The listing builds one solid part. Answer for the finished solid, in the listing's coordinates (mm). A direction names the side the tool comes from. Round coordinates to 2 decimals unless told otherwise and drop trailing zeros. Write each loop counter-clockwise with the first axis right and the second up, starting at its lowest first coordinate (ties: lowest second). Pieces come first, ordered by that corner, then holes. Notation, with made-up numbers: (-36, 32) - (-21, 32) arc R21 ccw to (-21, 46) - close; hole circle Ø1 at (70, 23). An arc over 180 degrees is marked (long way). Answer as CSV lines item,"result". Start each with the question number.
Item 1: Which of the six approach directions +Z, -Z, +X, -X, +Y, -Y give full straight-line access (tool end or side, diameter ignored) to faces 4 (the cylindrical face through (-0.54, 3.37, 2.44)), 5 (the flat face through (-1.293, -1.958, 0.76)), 6 (the flat face through (2, -3.1, 0))?
Item 2: Flat-ended cylindrical pins translate along their axes: pin 1 (5 mm diameter, centred on y = 2, z = 0, fed in from -X); pin 2 (1.5 mm diameter, centred on y = 2.5, z = 1, fed in from +X); pin 3 (4 mm diameter, centred on x = -3, y = 0, fed in from -Z). Find the tip coordinate at first contact, or state that the pin passes through.
Item 3: A cutting plane is placed at B-B on y = -0.5. Determine the outline of the cut face in (x, z).
Item 4: Straight lines are drawn through the part: line 1 along Z through (x, y) = (0, -1.5); line 2 along Y through (x, z) = (0.25, 2.25); line 3 along Z through (x, y) = (1.25, -1). For each, find the intervals that lie inside material, in ascending order. Write a range as [from, to].
Item 5: For a pull along Z with two mould halves and no side action, classify faces 1 (the flat face through (0, -2, -1.5)), 2 (the flat face through (0, 6.9, 0)), 3 (the conical face through (-0.351, -0.193, 2.671)) as pulls with the +Z half, pulls with the -Z half, needs draft (parallel to the pull), parting line crosses it, or undercut.
Item 6: A cutting plane is placed at A-A on y = 3.75. Determine the outline of the cut face in (x, z).
Solid Edge part; units mm, degrees
sketch "Sketch1" plane through (0, 0, 0) normal (0, 0, 1) x (1, 0, 0)
  line L0 (2.5, 0) -> (2.5, 6.9)
  line L1 (0, 6.9) -> (2.5, 6.9)
  line L2 (0, 0) -> (0, 6.9)
  line L3 (0, 0) -> (0, -3.1)
  line L4 (0, -3.1) -> (4.715, -3.1)
  line L5 (4.715, -3.1) -> (4.715, -2.215)
  line L6 (4.715, -2.215) -> (2.5, 0)
revolve "RevolvedProtrusion1" add sketch "Sketch1" angle 360 about axis through (0, 0, 0) along (0, 1, 0)
sketch "Sketch2" plane through (0, 0, 0) normal (1, 0, 0) x (0, 1, 0)
  line L0 (-3.1, 2.2215) -> (-1.2, 2.2215)
  line L1 (0.0826, 0) -> (-1.2, 2.2215)
  line L2 (-3.1, 0) -> (0.0826, 0)
  line L3 (-3.1, 0) -> (-3.1, 2.2215)
revolve "RevolvedCutout1" cut sketch "Sketch2" angle 360 about axis through (0, -4.5, 0) along (0, 1, 0)
sketch "Sketch3" plane through (0, -3.1, 0) normal (0, -1, 0) x (0, 0, 1)
  circle A0 centre (0, 0) radius 2.2215
  line L0 (-1.5, -0.866) -> (0, -1.7321)
  line L1 (0, -1.7321) -> (1.5, -0.866)
  line L2 (1.5, -0.866) -> (1.5, 0.866)
  line L3 (1.5, 0.866) -> (0, 1.7321)
  line L4 (0, 1.7321) -> (-1.5, 0.866)
  line L5 (-1.5, 0.866) -> (-1.5, -0.866)
extrude "Protrusion1" add sketch "Sketch3" against normal up to next
sketch "Sketch4" plane through (0, 0, 0) normal (0, 0, 1) x (1, 0, 0)
  line L0 (-1.7321, -3.1) -> (0, -3.1)
  line L1 (0, -3.1) -> (0, -2.6359)
  line L2 (0, -2.6359) -> (-1.7321, -3.1)
revolve "RevolvedCutout2" cut sketch "Sketch4" angle 360 about axis through (0, -4.5, 0) along (0, 1, 0)
fillet "Round1" radius 0.2 1 edges at (0, 0, -2.5)
chamfer "倒斜角_2" distance 0.3333 angle 45 1 edges at (0, 6.9, -2.5)
cosmetic_thread "Thread1"
properties part number "N2611-0314" material "铝 1060"
Geometry says:
1,face 4,"+Y"
1,face 5,"-Y"
1,face 6,"+Z, -Z, +X, -X, -Y"
2,pin 1,"stops at x = -3"
2,pin 2,"stops at x = 2.49"
2,pin 3,"stops at z = -3.74"
3,outline,"circle Ø6 at (0, 0); hole circle Ø2.02 at (0, 0)"
4,line 1,"z = [-4, -1.5], [1.5, 4]"
4,line 2,"y = [-3.1, 6.8]"
4,line 3,"z = [-3.27, -0.83], [0.83, 3.27]"
5,face 1,"undercut"
5,face 2,"needs draft"
5,face 3,"parting line crosses it"
6,outline,"circle Ø5 at (0, 0)"
